from build123d import *

# Parameters (mm, degrees)
BASPROSKE_W        = 4
BASPROSKE_H        = 9.5
TOOTHCUT_DEPTH     = 15.017845769
TEETHCUTS_COUNT    = 17
TEETHCUTS_ANGLE    = 338.823529412
BORSKE_R           = 0.4
BORE_DEPTH         = 50.0000508
CUT_EXTRUDE1_DEPTH = 15.003283988


with BuildPart() as part:
    # BasProSke → Base-Revolve (revolve)
    with BuildSketch(Plane(origin=(0, 0, 0), x_dir=(1, 0, 0), z_dir=(0, 1, 0)), mode=Mode.PRIVATE) as base_revolve_sk:
        with Locations((2, 4.75)):
            Rectangle(BASPROSKE_W, BASPROSKE_H)
    revolve(base_revolve_sk.sketch.rotate(Axis((-10, 0, 0), (1, 0, 0)), 180), axis=Axis((-10, 0, 0), (1, 0, 0)))

    # TooCutSke → ToothCut (cut, through all)
    with BuildSketch(Plane(origin=(0, 0, 0), x_dir=(0, 0, -1), z_dir=(1, 0, 0))):
        with BuildLine():
            ThreePointArc((0.516861231, 7.23055015), (0, 7.249), (-0.516861231, 7.23055015))
            ThreePointArc((-0.516861231, 7.23055015), (-0.827352654, 8.408398361), (-1.533069197, 9.401220346))
            ThreePointArc((-1.533069197, 9.401220346), (0, 9.5254), (1.533069197, 9.401220346))
            ThreePointArc((1.533069197, 9.401220346), (0.827352654, 8.408398361), (0.516861231, 7.23055015))
        make_face()
    toothcut = extrude(amount=TOOTHCUT_DEPTH, mode=Mode.SUBTRACT)

    # TeethCuts: ToothCut ×17 about axis
    teethcuts_axis = Axis((-10, 0, 0), (1, 0, 0))
    for i in range(1, TEETHCUTS_COUNT):
        add(toothcut.rotate(teethcuts_axis, i * TEETHCUTS_ANGLE / (TEETHCUTS_COUNT - 1)), mode=Mode.SUBTRACT)

    # BorSke → Bore (cut, symmetric)
    with BuildSketch(Plane(origin=(0, 0, 0), x_dir=(0, 0, -1), z_dir=(1, 0, 0))):
        with Locations(Location((0, 0, 0), (0, 0, 180))):
            Circle(BORSKE_R)
    extrude(amount=BORE_DEPTH, both=True, mode=Mode.SUBTRACT)

    # Sketch1 → Cut-Extrude1 (cut, through all)
    with BuildSketch(Plane(origin=(4, 0, 0), x_dir=(0, 0, -1), z_dir=(1, 0, 0))):
        Polygon((3.0022214, 0), (1.5011107, 2.6), (-1.5011107, 2.6), (-3.0022214, 0), (-1.5011107, -2.6), (1.5011107, -2.6), align=None)
    extrude(amount=-CUT_EXTRUDE1_DEPTH, mode=Mode.SUBTRACT)


solid = part.part
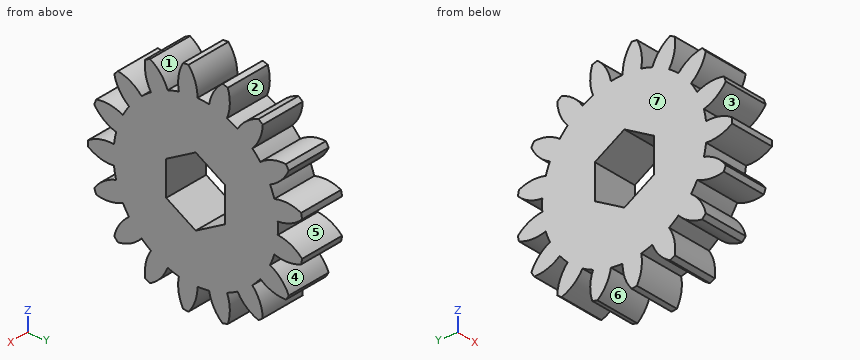
Could you check a few things on this model? Use its own coordinates, in mm. Face numbers are marked on the shaded views. A direction names the side the tool comes from. Give positions to 0.01 mm unless a question says otherwise; leave off trailing zeros. Order: outer loops, then holes, each group sorted by start corner. A loop starts at its lowest first (then second) coordinate and runs counter-clockwise, first axis right, second up. Notation, with made-up numbers: (73.5, -34) - (100.5, -34) arc R7 cw to (100.5, -25) - close; hole circle Ø11 at (3, 52.25). An arc over 180 degrees is marked (long way). Return JSON: item names as keys, results as strings. Group by question number.
Q1. Will this pin go through, and if not, where does the flat tip stop? pin 1 Ø1.5 at (y, z) = (0.5, -0.5) entering from +X.
Q2. Suppose I cut it at B-B, the plane y = -8. Please give me the cut outline in (x, z).
Q3. Please list where these lines run through material, in increasing order: line 1 along Z through (x, y) = (1.85, -6.5); line 2 along Y through (x, z) = (1.2, 8.25); line 3 along Z through (x, y) = (0.65, -7.25). Write a range as [from, to].
Q4. Which directions (+Z, -Z, +X, -X, +Y, -Y) give clear straight access to the entire face, cutting with the end or side of a thin tool? Please do the marked faces 1, 2, 3 and 4.
Q5. Suppose I cut it at A-A, the plane y = -0.25. Please give me the cut outline in (x, z), and give its area (3 significant figures).
Q6. Suppose I cut it at D-D, the plane y = 4.25. Please give me the cut outline in (x, z).
Q7. Thinking about a two-plate mould opening in Z: for the marked faces 5, 6 and 7, which applies, pulls with the +Z half, pulls with the -Z half, needs draft (parallel to the pull), parting line crosses it, or undercut?
Q8. Suppose I cut it at C-C, the plane y = -5. Please give me the cut outline in (x, z).
Resolved:
{
 "1": {"pin 1": "passes through"},
 "2": {"outline": "(0, -3.75) - (4, -3.75) - (4, -2.28) - (0, -2.28) - close; (0, -0.81) - (4, -0.81) - (4, 0.81) - (0, 0.81) - close; (0, 2.28) - (4, 2.28) - (4, 3.75) - (0, 3.75) - close"},
 "3": {"line 1": "z = [-6.51, -4.84], [-3.41, 3.41], [4.84, 6.51]", "line 2": "y = [-4.46, -3.49], [-1.52, 0.02], [1.57, 3]", "line 3": "z = [-3.67, -1.91], [-0.83, 0.83], [1.91, 3.67]"},
 "4": {"face 1": "+Z, +X, -X", "face 2": "+X, -X", "face 3": "+X, -X, -Y", "face 4": "+X, -X, +Y"},
 "5": {"outline": "(0, -8.9) - (4, -8.9) - (4, -2.86) - (0, -2.86) - close; (0, 2.86) - (4, 2.86) - (4, 8.9) - (0, 8.9) - close", "area": "48.4 mm2"},
 "6": {"outline": "(0, -6.95) - (4, -6.95) - (4, 6.95) - (0, 6.95) - close"},
 "7": {"face 5": "undercut", "face 6": "pulls with the -Z half", "face 7": "needs draft"},
 "8": {"outline": "(0, -5.69) - (4, -5.69) - (4, 5.69) - (0, 5.69) - close"}
}
